Can you work these out from the model? Positions are in its coordinate system, mm. A direction names the side the tool comes from. Round coordinates to 2 decimals unless told otherwise and drop trailing zeros. Loops run counter-clockwise (first coordinate to the right, second up) from the corner with the lowest first, then second, coordinate; pieces in that order, holes last.
```python
from build123d import *

# Parameters (mm, degrees)
SKETCH1_W           = 27.7
SKETCH1_H           = 24.3
BOSS_EXTRUDE1_DEPTH = 98.8
CHAMFER1_SIZE       = 5
CHAMFER2_SIZE       = 1.5
SKETCH2_W           = 13
SKETCH2_H           = 5
CUT_EXTRUDE1_DEPTH  = 15
SKETCH3_W           = 7
SKETCH3_H           = 2.4
CUT_EXTRUDE3_DEPTH  = 10
FILLET1_R           = 1.5


with BuildPart() as part:
    # Sketch1 → Boss-Extrude1 (new body)
    with BuildSketch(Plane.XY):
        with Locations((13.85, 12.15)):
            Rectangle(SKETCH1_W, SKETCH1_H)
    extrude(amount=BOSS_EXTRUDE1_DEPTH)

    # Chamfer1
    chamfer1_edges = [part.edges().sort_by_distance(p)[0] for p in [
        (0, 24.3, 49.4),
        (27.7, 24.3, 49.4),
        (27.7, 0, 49.4),
        (0, 0, 49.4),
    ]]
    chamfer(chamfer1_edges, length=CHAMFER1_SIZE)

    # Chamfer2
    chamfer2_edges = [part.edges().sort_by_distance(p)[0] for p in [
        (13.85, 24.3, 0),
        (13.85, 0, 0),
        (13.85, 24.3, 98.8),
        (13.85, 0, 98.8),
    ]]
    chamfer(chamfer2_edges, length=CHAMFER2_SIZE)

    # Sketch2 → Cut-Extrude1 (cut)
    with BuildSketch(Plane.XY.offset(98.8)):
        with Locations((13.7, 15.100435324)):
            Rectangle(SKETCH2_W, SKETCH2_H)
    extrude(amount=-CUT_EXTRUDE1_DEPTH, mode=Mode.SUBTRACT)

    # Sketch3 → Cut-Extrude3 (cut)
    with BuildSketch(Plane.XY.offset(98.8)):
        with Locations((13.85, 9.000435324)):
            Rectangle(SKETCH3_W, SKETCH3_H)
    extrude(amount=-CUT_EXTRUDE3_DEPTH, mode=Mode.SUBTRACT)

    # Fillet1
    fillet1_edges = [part.edges().sort_by_distance(p)[0] for p in [
        (10.35, 10.200435324, 93.8),
        (17.35, 10.200435324, 93.8),
    ]]
    fillet(fillet1_edges, radius=FILLET1_R)


solid = part.part
```
(1) Suppose I cut it at B-B (x = 18.5). Write out the boundary of the cut face in (y, z), then the cut area to 3 significant figures.
(2) For pin 1 (4 mm diameter, centred on x = 13, y = 15.5, fed in from +Z); pin 2 (4 mm diameter, centred on y = 21.5, z = 37.5, fed in from -X); pin 3 (1.9 mm diameter, centred on x = 14, y = 9, fed in from +Z); pin 4 (4 mm diameter, centred on y = 21, z = 46, fed in from -X), each with a flat end and sliding along its axis, tell me the tip position at first contact or that it passes through.
(3) We'd pull the mould along Y, two halves only. Please class faces 3 (the flat face through (25.2, 2.5, 48.7)), 4 (the flat face through (14, 12, 0)), 5 (the flat face through (20.2, 15, 91)): released by +Y, released by -Y, zero draft, split by the parting line, or undercut.
(4) Suppose I cut it at A-A (z = 85.5). Write out the boundary of the cut face in (x, y).
(5) Which directions (+Z, -Z, +X, -X, +Y, -Y) give clear straight access to the entire face, cutting with the end or side of a thin tool? Please do faces 1 (the flat face through (14, 24.3, 49)), 2 (the flat face through (14, 10.2, 94)).
(6) If I drill on line 1 (Y direction, x = 15.5, z = 90.5); line 2 (Y direction, x = 7.5, z = 87); line 3 (Y direction, x = 3.5, z = 73), over which ranges is the centre line in solid material (lowest first)?
(7) Suppose I cut it at C-C (y = 14). Write out the boundary of the cut face in (x, z).
(8) Suppose I cut it at D-D (z = 35). Write out the boundary of the cut face in (x, y), then the cut area to 3 significant figures.
Check result:
1. outline: (0, 1.5) - (1.5, 0) - (22.8, 0) - (24.3, 1.5) - (24.3, 97.3) - (22.8, 98.8) - (17.6, 98.8) - (17.6, 83.8) - (12.6, 83.8) - (12.6, 98.8) - (1.5, 98.8) - (0, 97.3) - close
1. area: 2,320 mm2
2. pin 1: stops at z = 83.8
2. pin 2: stops at x = 0.2
2. pin 3: stops at z = 88.8
2. pin 4: stops at x = 0
3. face 3: released by -Y
3. face 4: zero draft
3. face 5: undercut
4. outline: (0, 5) - (5, 0) - (22.7, 0) - (27.7, 5) - (27.7, 19.3) - (22.7, 24.3) - (5, 24.3) - (0, 19.3) - close; hole (7.2, 12.6) - (20.2, 12.6) - (20.2, 17.6) - (7.2, 17.6) - close
5. face 1: +Z, -Z, +X, -X, +Y
5. face 2: +Z
6. line 1: y = 0 to 7.8, 10.2 to 12.6, 17.6 to 24.3
6. line 2: y = 0 to 12.6, 17.6 to 24.3
6. line 3: y = 1.5 to 22.8
7. outline: (0, 0) - (27.7, 0) - (27.7, 98.8) - (20.2, 98.8) - (20.2, 83.8) - (7.2, 83.8) - (7.2, 98.8) - (0, 98.8) - close
8. outline: (0, 5) - (5, 0) - (22.7, 0) - (27.7, 5) - (27.7, 19.3) - (22.7, 24.3) - (5, 24.3) - (0, 19.3) - close
8. area: 623 mm2
